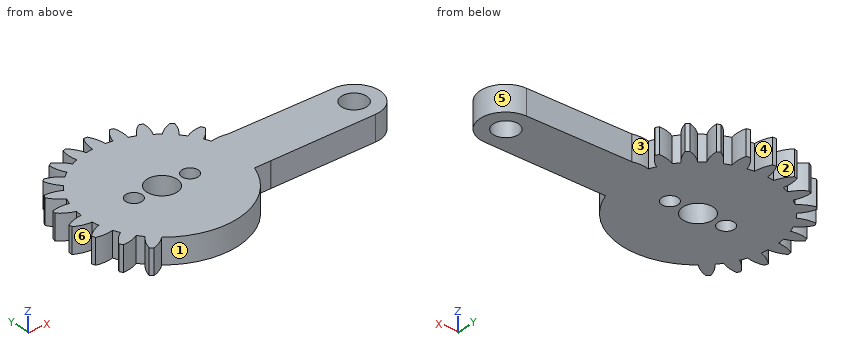
```python
from build123d import *

# Parameters (mm, degrees)
SKETCH1_R           = 12.09
SKETCH1_R_2         = 1.75
SKETCH1_R_3         = 1.995
BOSS_EXTRUDE1_DEPTH = 4
SKETCH2_R           = 1.3
SKETCH2_R_2         = 2.4
CUT_EXTRUDE1_DEPTH  = 38.96437919


with BuildPart() as part:
    # Sketch1 → Boss-Extrude1 (new body)
    # profile 1 of 22: a face of its own
    with BuildSketch(Plane.XY):
        Circle(SKETCH1_R)
        Circle(SKETCH1_R_2, mode=Mode.SUBTRACT)
    # profile 2 of 22: a face of its own
    with BuildSketch(Plane.XY):
        with BuildLine():
            ThreePointArc((14.051469909, -4.073462091), (14.048317136, -4.084321933), (14.04515597, -4.095179336))
            Line((14.04515597, -4.095179336), (30.82582707, -3.999919373))
            ThreePointArc((30.82582707, -3.999919373), (34.803112279, -0.008027822), (30.841914591, 3.999828048))
            Line((30.841914591, 3.999828048), (14.04515597, 4.095179336))
            ThreePointArc((14.04515597, 4.095179336), (14.128586435, 3.797360314), (14.205702589, 3.497844187))
            ThreePointArc((14.205702589, 3.497844187), (14.50484412, 1.909554151), (14.626965513, 0.297959519))
            ThreePointArc((14.626965513, 0.297959519), (14.629241359, 0.148987485), (14.63, 0))
            ThreePointArc((14.63, 0), (14.629241116, -0.149011314), (14.626964543, -0.298007168))
            ThreePointArc((14.626964543, -0.298007168), (14.504858624, -1.909443973), (14.20576712, -3.497582099))
            ThreePointArc((14.20576712, -3.497582099), (14.131552306, -3.786308154), (14.051469909, -4.073462091))
        make_face()
        with Locations((30.75, 0)):
            Circle(SKETCH1_R_3, mode=Mode.SUBTRACT)
    # profile 3 of 22: a face of its own
    with BuildSketch(Plane.XY):
        with BuildLine():
            ThreePointArc((14.205702589, 3.497844187), (14.128586435, 3.797360314), (14.04515597, 4.095179336))
            Line((14.04515597, 4.095179336), (13.966164937, 4.095627749))
            Line((13.966164937, 4.095627749), (11.369827915, 4.11036655))
            ThreePointArc((11.369827915, 4.11036655), (11.678097516, 3.128919686), (11.901816808, 2.124819208))
            ThreePointArc((11.901816808, 2.124819208), (13.1403578, 2.666023245), (14.205702589, 3.497844187))
        make_face()
    # profile 4 of 22: a face of its own
    with BuildSketch(Plane.XY):
        with BuildLine():
            ThreePointArc((-12.517636695, -7.572692492), (-11.175984377, -7.407777173), (-9.917325106, -6.914821961))
            ThreePointArc((-9.917325106, -6.914821961), (-10.469253219, -6.046721181), (-10.945386333, -5.134843524))
            ThreePointArc((-10.945386333, -5.134843524), (-12.001489862, -5.978375477), (-12.815033037, -7.057749518))
            ThreePointArc((-12.815033037, -7.057749518), (-12.668951436, -7.31673216), (-12.517636695, -7.572692492))
        make_face()
    # profile 5 of 22: a face of its own
    with BuildSketch(Plane.XY):
        with BuildLine():
            ThreePointArc((-14.051145033, -4.074582586), (-12.712516328, -4.262616236), (-11.369129658, -4.112297512))
            ThreePointArc((-11.369129658, -4.112297512), (-11.677558471, -3.130930876), (-11.901445615, -2.126897335))
            ThreePointArc((-11.901445615, -2.126897335), (-13.139881298, -2.668425004), (-14.205038564, -3.500539874))
            ThreePointArc((-14.205038564, -3.500539874), (-14.13100701, -3.788342761), (-14.051145033, -4.074582586))
        make_face()
    # profile 6 of 22: a face of its own
    with BuildSketch(Plane.XY):
        with BuildLine():
            ThreePointArc((-14.626950262, -0.298707293), (-13.382615157, -0.826868574), (-12.046093246, -1.029435529))
            ThreePointArc((-12.046093246, -1.029435529), (-12.089999882, -0.001686428), (-12.046379968, 1.026074882))
            ThreePointArc((-12.046379968, 1.026074882), (-13.382791491, 0.823465153), (-14.62701917, 0.295313712))
            ThreePointArc((-14.62701917, 0.295313712), (-14.629999902, -0.00169714), (-14.626950262, -0.298707293))
        make_face()
    # profile 7 of 22: a face of its own
    with BuildSketch(Plane.XY):
        with BuildLine():
            ThreePointArc((-14.205774364, 3.497552675), (-13.140565234, 2.66528054), (-11.902026335, 2.123645243))
            ThreePointArc((-11.902026335, 2.123645243), (-11.678416405, 3.127729251), (-11.370260409, 4.109170017))
            ThreePointArc((-11.370260409, 4.109170017), (-12.71360248, 4.259309779), (-14.052145793, 4.071129894))
            ThreePointArc((-14.052145793, 4.071129894), (-14.131870386, 3.78512079), (-14.205774364, 3.497552675))
        make_face()
    # profile 8 of 22: a face of its own
    with BuildSketch(Plane.XY):
        with BuildLine():
            ThreePointArc((-9.919135011, 6.912225448), (-11.177872267, 7.404913556), (-12.519533027, 7.569556974))
            ThreePointArc((-12.519533027, 7.569556974), (-12.670533379, 7.313992337), (-12.816317544, 7.055416686))
            ThreePointArc((-12.816317544, 7.055416686), (-12.00284137, 5.975783406), (-10.94671211, 5.132016561))
            ThreePointArc((-10.94671211, 5.132016561), (-10.470825179, 6.043998682), (-9.919135011, 6.912225448))
        make_face()
    # profile 9 of 22: a face of its own
    with BuildSketch(Plane.XY):
        with BuildLine():
            ThreePointArc((-7.791898403, 9.244155952), (-8.880242473, 10.045843984), (-10.13359017, 10.552120653))
            ThreePointArc((-10.13359017, 10.552120653), (-10.345575707, 10.344368676), (-10.553302948, 10.1323589))
            ThreePointArc((-10.553302948, 10.1323589), (-10.04699158, 8.878969486), (-9.245249077, 7.790601357))
            ThreePointArc((-9.245249077, 7.790601357), (-8.549520677, 8.54832125), (-7.791898403, 9.244155952))
        make_face()
    # profile 10 of 22: a face of its own
    with BuildSketch(Plane.XY):
        with BuildLine():
            ThreePointArc((-5.133551517, 10.945992364), (-5.977311447, 12.002061971), (-7.05691548, 12.815492339))
            ThreePointArc((-7.05691548, 12.815492339), (-7.315469666, 12.669680484), (-7.571012334, 12.518652972))
            ThreePointArc((-7.571012334, 12.518652972), (-7.40634855, 11.176941958), (-6.913615931, 9.918165897))
            ThreePointArc((-6.913615931, 9.918165897), (-6.045466706, 10.469977665), (-5.133551517, 10.945992364))
        make_face()
    # profile 11 of 22: a face of its own
    with BuildSketch(Plane.XY):
        with BuildLine():
            ThreePointArc((-2.125311093, 11.901728982), (-2.666957342, 13.14020836), (-3.499215334, 14.205364904))
            ThreePointArc((-3.499215334, 14.205364904), (-3.786765286, 14.131429817), (-4.072755654, 14.051674682))
            ThreePointArc((-4.072755654, 14.051674682), (-4.260931239, 12.713077321), (-4.110760617, 11.369685446))
            ThreePointArc((-4.110760617, 11.369685446), (-3.129363382, 11.677978627), (-2.125311093, 11.901728982))
        make_face()
    # profile 12 of 22: a face of its own
    with BuildSketch(Plane.XY):
        with BuildLine():
            ThreePointArc((1.027754616, 12.046236775), (0.825159863, 13.382704508), (0.296996585, 14.626985097))
            ThreePointArc((0.296996585, 14.626985097), (0, 14.63), (-0.296996585, 14.626985097))
            ThreePointArc((-0.296996585, 14.626985097), (-0.825159863, 13.382704508), (-1.027754616, 12.046236775))
            ThreePointArc((-1.027754616, 12.046236775), (0, 12.09), (1.027754616, 12.046236775))
        make_face()
    # profile 13 of 22: a face of its own
    with BuildSketch(Plane.XY):
        with BuildLine():
            ThreePointArc((4.110717434, 11.369701059), (4.260994095, 12.713043392), (4.072942889, 14.051620413))
            ThreePointArc((4.072942889, 14.051620413), (3.786710214, 14.131444574), (3.498915331, 14.2054388))
            ThreePointArc((3.498915331, 14.2054388), (2.666773966, 13.14023428), (2.125244746, 11.901740829))
            ThreePointArc((2.125244746, 11.901740829), (3.129308654, 11.677993293), (4.110717434, 11.369701059))
        make_face()
    # profile 14 of 22: a face of its own
    with BuildSketch(Plane.XY):
        with BuildLine():
            ThreePointArc((6.913450185, 9.91828143), (7.406352802, 11.176909529), (7.571236986, 12.518517105))
            ThreePointArc((7.571236986, 12.518517105), (7.315275528, 12.669792577), (7.056292749, 12.81583523))
            ThreePointArc((7.056292749, 12.81583523), (5.976880257, 12.002254067), (5.133331053, 10.946095756))
            ThreePointArc((5.133331053, 10.946095756), (6.045273784, 10.470089058), (6.913450185, 9.91828143))
        make_face()
    # profile 15 of 22: a face of its own
    with BuildSketch(Plane.XY):
        with BuildLine():
            ThreePointArc((9.244954117, 7.790951378), (10.046869152, 8.879052728), (10.553440202, 10.132215942))
            ThreePointArc((10.553440202, 10.132215942), (10.345229175, 10.344715236), (10.132740224, 10.552936821))
            ThreePointArc((10.132740224, 10.552936821), (8.879594749, 10.046380548), (7.791503622, 9.244488699))
            ThreePointArc((7.791503622, 9.244488699), (8.549176321, 8.548665641), (9.244954117, 7.790951378))
        make_face()
    # profile 16 of 22: a face of its own
    with BuildSketch(Plane.XY):
        with BuildLine():
            ThreePointArc((10.946374382, 5.132736881), (12.002615026, 5.976132183), (12.81632055, 7.055411226))
            ThreePointArc((12.81632055, 7.055411226), (12.670115094, 7.314716911), (12.518663963, 7.570994161))
            ThreePointArc((12.518663963, 7.570994161), (11.17714698, 7.405952739), (9.918639175, 6.912936924))
            ThreePointArc((9.918639175, 6.912936924), (10.47040953, 6.044718709), (10.946374382, 5.132736881))
        make_face()
    # profile 17 of 22: a face of its own
    with BuildSketch(Plane.XY):
        with BuildLine():
            ThreePointArc((12.046231207, -1.027819886), (11.986581537, -1.577961676), (11.901820644, -2.124797724))
            ThreePointArc((11.901820644, -2.124797724), (13.140374441, -2.665881604), (14.20576712, -3.497582099))
            ThreePointArc((14.20576712, -3.497582099), (14.504858624, -1.909443973), (14.626964543, -0.298007168))
            ThreePointArc((14.626964543, -0.298007168), (13.382627003, -0.825679814), (12.046231207, -1.027819886))
        make_face()
    # profile 18 of 22: a face of its own
    with BuildSketch(Plane.XY):
        with BuildLine():
            ThreePointArc((11.901820644, -2.124797724), (11.67810034, -3.128909147), (11.369827915, -4.11036655))
            Line((11.369827915, -4.11036655), (13.967019497, -4.095622898))
            ThreePointArc((13.967019497, -4.095622898), (14.009289492, -4.084713176), (14.051469909, -4.073462091))
            ThreePointArc((14.051469909, -4.073462091), (14.131552306, -3.786308154), (14.20576712, -3.497582099))
            ThreePointArc((14.20576712, -3.497582099), (13.140374441, -2.665881604), (11.901820644, -2.124797724))
        make_face()
    # profile 19 of 22: a face of its own
    with BuildSketch(Plane.XY):
        with BuildLine():
            ThreePointArc((12.09, 0), (12.079052845, -0.514375696), (12.046231207, -1.027819886))
            ThreePointArc((12.046231207, -1.027819886), (13.382627003, -0.825679814), (14.626964543, -0.298007168))
            ThreePointArc((14.626964543, -0.298007168), (14.629241116, -0.149011314), (14.63, 0))
            ThreePointArc((14.63, 0), (14.629241359, 0.148987485), (14.626965513, 0.297959519))
            ThreePointArc((14.626965513, 0.297959519), (13.382629481, 0.825632028), (12.046235232, 1.027772701))
            ThreePointArc((12.046235232, 1.027772701), (12.079053853, 0.514352039), (12.09, 0))
        make_face()
    # profile 20 of 22: a face of its own
    with BuildSketch(Plane.XY):
        with BuildLine():
            ThreePointArc((11.901816808, 2.124819208), (11.986583203, 1.577949019), (12.046235232, 1.027772701))
            ThreePointArc((12.046235232, 1.027772701), (13.382629481, 0.825632028), (14.626965513, 0.297959519))
            ThreePointArc((14.626965513, 0.297959519), (14.50484412, 1.909554151), (14.205702589, 3.497844187))
            ThreePointArc((14.205702589, 3.497844187), (13.1403578, 2.666023245), (11.901816808, 2.124819208))
        make_face()
    # profile 21 of 22: a face of its own
    with BuildSketch(Plane.XY):
        with BuildLine():
            Line((11.369827915, 4.11036655), (13.966164937, 4.095627749))
            ThreePointArc((13.966164937, 4.095627749), (12.668895431, 4.261362771), (11.369827915, 4.11036655))
        make_face()
    # profile 22 of 22: a face of its own
    with BuildSketch(Plane.XY):
        with BuildLine():
            ThreePointArc((-10.130994605, -10.554612656), (-8.877796666, -10.047999865), (-7.789679206, -9.246026058))
            ThreePointArc((-7.789679206, -9.246026058), (-8.547489799, -8.550351931), (-9.243417598, -7.792774288))
            ThreePointArc((-9.243417598, -7.792774288), (-10.045261463, -8.880834456), (-10.55179143, -10.133932978))
            ThreePointArc((-10.55179143, -10.133932978), (-10.343531911, -10.346412306), (-10.130994605, -10.554612656))
        make_face()
    extrude(amount=BOSS_EXTRUDE1_DEPTH)

    # Sketch2 → Cut-Extrude1 (cut, through all)
    with BuildSketch(Plane.XY.offset(4)):
        with Locations((4.5, 0)):
            Circle(SKETCH2_R)
        with Locations((-4.5, 0)):
            Circle(SKETCH2_R)
        Circle(SKETCH2_R_2)
    extrude(amount=-CUT_EXTRUDE1_DEPTH, mode=Mode.SUBTRACT)


solid = part.part
```
Input: part model. Units: mm. Frame: model coordinates. Face numbers are marked on the shaded views. A direction names the side the tool comes from. Coordinates: 2 decimals unless noted, no trailing zeros. Write each loop counter-clockwise with the first axis right and the second up, starting at its lowest first coordinate (ties: lowest second). Pieces come first, ordered by that corner, then holes.
1) Set-up query: the marked faces 1, 2 and 3. Return all of +Z, -Z, +X, -X, +Y, -Y with unobstructed straight access to the full face (end or side cutting, diameter ignored); none if empty.
2) Section A-A on z = 2.2. State how many separate pieces and enclosed holes the cut face has, and give its area (3 significant figures).
3) Material intervals for line 1 along Y through (x, z) = (0, 2.9); line 2 along X through (y, z) = (13, 2.2); line 3 along X through (y, z) = (-0.5, 0.65), sorted ascending.
4) Section B-B on x = 27.5. Output: boundary loops of the cut face in (y, z), and give its area (3 significant figures).
5) Section C-C on x = 19. Output: boundary loops of the cut face in (y, z).
6) Mould query, pull axis X, two halves, no side actions, for the marked faces 4, 5 and 6. Classes: pulls with the +X half, pulls with the -X half, needs draft (parallel to the pull), parting line crosses it, or undercut.
7) Pin query (flat end, axial travel): pin 1 Ø1 at (x, z) = (19.5, 2.5) entering from +Y; pin 2 Ø2 at (y, z) = (8, 1.5) entering from +X. Return the tip coordinate at first contact, or that it passes through.
Check result:
1. face 1: +Z, -Z, -Y
1. face 2: +Z, -Z, +Y
1. face 3: +Z, -Z
2. separate pieces: 1
2. enclosed holes: 4
2. area: 653 mm2
3. line 1: y = -12.09 to -2.4, 2.4 to 14.63
3. line 2: x = -4.25 to -2.59, -0.92 to 0.92, 2.59 to 4.25
3. line 3: x = -14.25 to -5.7, -3.3 to -2.35, 2.35 to 3.3, 5.7 to 28.82, 32.68 to 34.77
4. outline: (-4.02, 0) - (4.02, 0) - (4.02, 4) - (-4.02, 4) - close
4. area: 32.2 mm2
5. outline: (-4.07, 0) - (4.07, 0) - (4.07, 4) - (-4.07, 4) - close
6. face 4: undercut
6. face 5: pulls with the +X half
6. face 6: pulls with the -X half
7. pin 1: stops at y = 4.07
7. pin 2: stops at x = 12.82
